Build history of the part. All positions in model axes, mm. Give positions to 0.01 mm unless a question says otherwise; leave off trailing zeros. Loops run counter-clockwise (first coordinate to the right, second up) from the corner with the lowest first, then second, coordinate; pieces in that order, holes last. Notation, with made-up numbers: M -29,43 L -24,43 A16 ccw -24,68 Z; hole C 68.25,4.5 d3. An arc over 180 degrees is marked long. Answer as a JSON object with one key per item and string values. Group by question number.
1. Slice it at A-A (z = 53.5). List the corners of the cut face in (x, y), then the cut area to 3 significant figures.
2. Drop flat-ended pins along their axis: pin 1 Ø4 at (x, z) = (38.5, -69.5) entering from -Y; pin 2 Ø1 at (x, z) = (23, -104.5) entering from -Y; pin 3 Ø3 at (x, y) = (13, -1565.5) entering from +Z. Give the stop position or say it passes through.
3. Slice it at B-B (x = -34). List the corners of the cut face in (y, z), then the cut area to 3 significant figures.
4. Drill centre lines: line 1 along Z through (x, y) = (141, -1566); line 2 along Y through (x, z) = (9.5, -71.5); line 3 along X through (y, z) = (-1567.25, -17). Where is each one in solid material? Low to high. Write a range as [from, to].
5. Mould opens along X. For faces 1 (the face through (266.49, -1564.58, -125.13)), 2 (the face through (209, -1566.1, 11.3)) say: released by +X, released by -X, zero draft, split by the parting line, or undercut.
from build123d import *

# Parameters (mm, degrees)
BOSS_EXTRUDE1_DEPTH = 3.175
SKETCH4_R           = 20.32
CUT_EXTRUDE1_DEPTH  = 3.175


with BuildPart() as part:
    # Sketch1 → Boss-Extrude1 (new body)
    with BuildSketch(Plane(origin=(3.144869288, -1568.333107971, -7.514232815), x_dir=(0.9999919583187062, 0.004010352693004623, 1.921449190373677e-05), z_dir=(-0.004010352693004623, 0.9999460479318565, 0.009582186427904116))):
        with BuildLine():
            Line((253.440636473, 121.814232815), (-104.805130712, 121.814232815))
            ThreePointArc((-104.805130712, 121.814232815), (-109.295258773, 119.954360876), (-111.155130712, 115.464232815))
            Line((-111.155130712, 115.464232815), (-111.155130712, -87.735767185))
            ThreePointArc((-111.155130712, -87.735767185), (-109.295258773, -92.225895245), (-104.805130712, -94.085767185))
            Line((-104.805130712, -94.085767185), (233.014869288, -94.085767185))
            ThreePointArc((233.014869288, -94.085767185), (237.504997348, -92.225895245), (239.364869288, -87.735767185))
            Line((239.364869288, -87.735767185), (239.364869288, 8.89))
            ThreePointArc((239.364869288, 8.89), (241.224741227, 13.380128061), (245.714869288, 15.24))
            Line((245.714869288, 15.24), (260.954869288, 15.24))
            ThreePointArc((260.954869288, 15.24), (265.444997348, 17.099871939), (267.304869288, 21.59))
            Line((267.304869288, 21.59), (267.304869288, 107.95))
            ThreePointArc((267.304869288, 107.95), (263.244129512, 117.753493039), (253.440636473, 121.814232815))
        make_face()
    extrude(amount=BOSS_EXTRUDE1_DEPTH)

    # Sketch4 → Cut-Extrude1 (cut)
    with BuildSketch(Plane(origin=(3.157601814, -1568.332765376, -7.544655436), x_dir=(0.9999919583187062, 0.004010352693004624, 1.9214491903792285e-05), z_dir=(-0.004010352693004624, 0.9999460479318565, 0.009582186427904121))):
        with Locations(Location((199.747601441, 0.556803893, 0), (0, 0, 269.998899082))):
            Circle(SKETCH4_R)
    extrude(amount=CUT_EXTRUDE1_DEPTH, mode=Mode.SUBTRACT)


solid = part.part
Established:
{
 "1": {"outline": "M -108.02,-1566.19 L -108.01,-1569.36 L 242.51,-1567.96 L 242.5,-1564.78 Z", "area": "1,110 mm^2"},
 "2": {"pin 1": "stops at y = -1567.62", "pin 2": "stops at y = -1567.33", "pin 3": "stops at z = 86.6"},
 "3": {"outline": "M -1569.38,86.57 L -1567.31,-129.32 L -1564.14,-129.29 L -1566.21,86.6 Z", "area": "685 mm^2"},
 "4": {"line 1": "z = [-129.31, 86.6]", "line 2": "y = [-1567.69, -1564.52]", "line 3": "x = [-108.02, 184.64], [221.17, 242.54]"},
 "5": {"face 1": "released by +X", "face 2": "undercut"}
}
